```python
from build123d import *

# Parameters (mm, degrees)
SKETCH1_W           = 690.5625
SKETCH1_H           = 320.675
SKETCH1_W_2         = 639.7625
SKETCH1_H_2         = 269.875
SKETCH1_W_3         = 25.4
SKETCH1_W_4         = 79.375
SKETCH1_H_3         = 25.4
BOSS_EXTRUDE1_DEPTH = 617.22
SKETCH2_W           = 566.42
SKETCH2_H           = 269.875
CUT_EXTRUDE1_DEPTH  = 981.137516082
BOSS_EXTRUDE2_DEPTH = 566.42
CUT_EXTRUDE2_REACH  = 741.293
SKETCH6_W           = 566.42
SKETCH6_H           = 79.375
SKETCH7_W           = 127
SKETCH7_H           = 203.2
SKETCH7_W_2         = 261.62
CUT_EXTRUDE3_DEPTH  = 773.950070043
CUT_EXTRUDE4_REACH  = 785.005
SKETCH8_W           = 566.42
SKETCH8_H           = 307.975
CUT_EXTRUDE6_REACH  = 785.005
SKETCH9_W           = 159.433185108
SKETCH9_H           = 305.57390625
SKETCH9_W_2         = 381.586814892
CUT_EXTRUDE8_REACH  = 774.95
SKETCH10_W          = 566.42
SKETCH10_H          = 306.3875
CUT_EXTRUDE10_REACH = 774.95
SKETCH12_W          = 566.42
SKETCH12_H          = 79.375
SKETCH13_W          = 617.22
SKETCH13_H          = 333.375
CUT_EXTRUDE13_DEPTH = 25.4


with BuildPart() as part:
    # Sketch1 → Boss-Extrude1 (new body)
    # profile 1 of 4: a face of its own
    with BuildSketch(Plane(origin=(0, 0, 0), x_dir=(0, 0, -1), z_dir=(1, 0, 0))):
        with Locations((-14.30734375, -160.3375)):
            Rectangle(SKETCH1_W, SKETCH1_H)
        with Locations((-14.30734375, -160.3375)):
            Rectangle(SKETCH1_W_2, SKETCH1_H_2, mode=Mode.SUBTRACT)
    # profile 2 of 4: a face of its own
    with BuildSketch(Plane(origin=(0, 0, 0), x_dir=(0, 0, -1), z_dir=(1, 0, 0))):
        Polygon((-0.81359375, -25.4), (-26.21359375, -25.4), (-26.21359375, -190.5), (-26.21359375, -215.9), (-26.21359375, -295.275), (-0.81359375, -295.275), align=None)
    # profile 3 of 4: a face of its own
    with BuildSketch(Plane(origin=(0, 0, 0), x_dir=(0, 0, -1), z_dir=(1, 0, 0))):
        with Locations((-118.28859375, -160.3375)):
            Rectangle(SKETCH1_W_3, SKETCH1_H_2)
    # profile 4 of 4: a face of its own
    with BuildSketch(Plane(origin=(0, 0, 0), x_dir=(0, 0, -1), z_dir=(1, 0, 0))):
        with Locations((-65.90109375, -203.2)):
            Rectangle(SKETCH1_W_4, SKETCH1_H_3)
    extrude(amount=BOSS_EXTRUDE1_DEPTH)

    # Sketch2 → Cut-Extrude1 (cut, through all)
    with BuildSketch(Plane.XY.offset(359.58859375)):
        with Locations((308.61, -160.3375)):
            Rectangle(SKETCH2_W, SKETCH2_H)
    extrude(amount=-CUT_EXTRUDE1_DEPTH, mode=Mode.SUBTRACT)

    # Sketch4 → Boss-Extrude2 (add)
    with BuildSketch(Plane(origin=(25.4, 0, 0), x_dir=(0, 0, -1), z_dir=(1, 0, 0))):
        Polygon((-26.21359375, -190.5), (-0.81359375, -190.5), (-0.81359375, -215.87774991), (-130.98859375, -215.87774991), (-130.98859375, -190.5), align=None)
    extrude(amount=BOSS_EXTRUDE2_DEPTH)

    # Sketch6 → Cut-Extrude2 (cut, up to next)
    with BuildSketch(Plane(origin=(0, -190.5, 0), x_dir=(1, 0, 0), z_dir=(0, 1, 0)), mode=Mode.PRIVATE) as cut_extrude2_sk1:
        with Locations((308.61, -65.90109375)):
            Rectangle(SKETCH6_W, SKETCH6_H)
    cut_extrude2_tool1 = extrude(cut_extrude2_sk1.sketch, amount=-CUT_EXTRUDE2_REACH, mode=Mode.PRIVATE) & part.part
    add(cut_extrude2_tool1.solids().sort_by_distance((308.61, -190.5, 65.901094))[0], mode=Mode.SUBTRACT)

    # Sketch7 → Cut-Extrude3 (cut, through all)
    with BuildSketch(Plane(origin=(0, -295.275, 0), x_dir=(1, 0, 0), z_dir=(0, 1, 0))):
        with Locations((528.32, -232.58859375)):
            Rectangle(SKETCH7_W, SKETCH7_H)
        with Locations((88.9, -232.58859375)):
            Rectangle(SKETCH7_W, SKETCH7_H)
        with Locations((308.61, -232.58859375)):
            Rectangle(SKETCH7_W_2, SKETCH7_H)
    extrude(amount=-CUT_EXTRUDE3_DEPTH, mode=Mode.SUBTRACT)

    # Sketch8 → Cut-Extrude4 (cut, up to next)
    with BuildSketch(Plane(origin=(0, 0, 0), x_dir=(1, 0, 0), z_dir=(0, 1, 0)), mode=Mode.PRIVATE) as cut_extrude4_sk1:
        with Locations((308.61, -180.20109375)):
            Rectangle(SKETCH8_W, SKETCH8_H)
    cut_extrude4_tool1 = extrude(cut_extrude4_sk1.sketch, amount=-CUT_EXTRUDE4_REACH, mode=Mode.PRIVATE) & part.part
    add(cut_extrude4_tool1.solids().sort_by_distance((308.61, 0, 180.201094))[0], mode=Mode.SUBTRACT)

    # Sketch9 → Cut-Extrude6 (cut, up to next)
    with BuildSketch(Plane(origin=(0, 0, 0), x_dir=(1, 0, 0), z_dir=(0, 1, 0)), mode=Mode.PRIVATE) as cut_extrude6_sk1:
        with Locations((105.116592554, 152.786953125)):
            Rectangle(SKETCH9_W, SKETCH9_H)
    cut_extrude6_tool1 = extrude(cut_extrude6_sk1.sketch, amount=-CUT_EXTRUDE6_REACH, mode=Mode.PRIVATE) & part.part
    # Sketch9 → Cut-Extrude6 (cut, up to next)
    with BuildSketch(Plane(origin=(0, 0, 0), x_dir=(1, 0, 0), z_dir=(0, 1, 0)), mode=Mode.PRIVATE) as cut_extrude6_sk2:
        with Locations((401.026592554, 152.786953125)):
            Rectangle(SKETCH9_W_2, SKETCH9_H)
    cut_extrude6_tool2 = extrude(cut_extrude6_sk2.sketch, amount=-CUT_EXTRUDE6_REACH, mode=Mode.PRIVATE) & part.part
    add(cut_extrude6_tool1.solids().sort_by_distance((105.116593, 0, -152.786953))[0], mode=Mode.SUBTRACT)
    add(cut_extrude6_tool2.solids().sort_by_distance((401.026593, 0, -152.786953))[0], mode=Mode.SUBTRACT)

    # Sketch10 → Cut-Extrude8 (cut, up to next)
    with BuildSketch(Plane(origin=(0, -295.275, 0), x_dir=(1, 0, 0), z_dir=(0, 1, 0)), mode=Mode.PRIVATE) as cut_extrude8_sk1:
        with Locations((308.61, 152.38015625)):
            Rectangle(SKETCH10_W, SKETCH10_H)
    cut_extrude8_tool1 = extrude(cut_extrude8_sk1.sketch, amount=-CUT_EXTRUDE8_REACH, mode=Mode.PRIVATE) & part.part
    add(cut_extrude8_tool1.solids().sort_by_distance((308.61, -295.275, -152.380156))[0], mode=Mode.SUBTRACT)

    # Sketch12 → Cut-Extrude10 (cut, up to next)
    with BuildSketch(Plane(origin=(0, -295.275, 0), x_dir=(1, 0, 0), z_dir=(0, 1, 0)), mode=Mode.PRIVATE) as cut_extrude10_sk1:
        with Locations((308.61, -65.90109375)):
            Rectangle(SKETCH12_W, SKETCH12_H)
    cut_extrude10_tool1 = extrude(cut_extrude10_sk1.sketch, amount=-CUT_EXTRUDE10_REACH, mode=Mode.PRIVATE) & part.part
    add(cut_extrude10_tool1.solids().sort_by_distance((308.61, -295.275, 65.901094))[0], mode=Mode.SUBTRACT)

    # Sketch13 → Cut-Extrude13 (cut)
    with BuildSketch(Plane(origin=(0, 0, 0), x_dir=(1, 0, 0), z_dir=(0, 1, 0))):
        with Locations((308.61, -192.90109375)):
            Rectangle(SKETCH13_W, SKETCH13_H)
    extrude(amount=-CUT_EXTRUDE13_DEPTH, mode=Mode.SUBTRACT)


solid = part.part
```
Check sheet for the modelled part. Datum: model origin and axes. Units: mm. A direction names the side the tool comes from. Coordinates: 2 decimals unless noted, no trailing zeros. Loops run counter-clockwise (first coordinate to the right, second up) from the corner with the lowest first, then second, coordinate; pieces in that order, holes last.
1) Sectioned sample at A-A (z = -153). Record the boundary of the cut face in (x, y) (3 decimals).
2) Access from +Z, -Z, +X, -X, +Y, -Y to the whole of each face (thin tool, end or side, straight path). Record for faces 1 (the face through (184.833, -13, -151)), 2 (the face through (591.82, -207, 67)), 3 (the face through (604, -295.275, 66)).
3) Sectioned sample at B-B (y = -155). Count the separate pieces of the cut face and the enclosed holes in it, and give its area (3 significant figures).
4) Gauge pin test, flat end, axial feed: pin 1 (12.5 mm diameter, centred on x = 16.5, z = 74.5, fed in from +Y). Record the tip position at first contact, or that the pin passes through.
5) Release check for a two-part mould opening along Z. For faces 4 (the face through (591.82, -308, 234)), 5 (the face through (604, -162, -305.574)), 6 (the face through (13, -25.4, 118)) record: released by +Z, released by -Z, zero draft, split by the parting line, or undercut.
6) Sectioned sample at C-C (z = 95.5). Record the boundary of the cut face in (x, y) (3 decimals).
7) Material ranges on probe 1 along Z at (x, y) = (360, -299); probe 2 along Z at (x, y) = (29.5, -197.5); probe 3 along Y at (x, z) = (438, 22) (3 decimals), recorded low to high.
Check sheet entries:
1. outline: (0, -320.675) - (25.4, -320.675) - (25.4, -295.275) - (0, -295.275) - close; (0, -25.4) - (25.4, -25.4) - (25.4, 0) - (0, 0) - close; (184.833, -25.4) - (210.233, -25.4) - (210.233, 0) - (184.833, 0) - close; (591.82, -320.675) - (617.22, -320.675) - (617.22, -295.275) - (591.82, -295.275) - close; (591.82, -25.4) - (617.22, -25.4) - (617.22, 0) - (591.82, 0) - close
2. face 1: +Y, -Y
2. face 2: none
2. face 3: +X, -X
3. separate pieces: 8
3. enclosed holes: 0
3. area: 5,160 mm2
4. pin 1: stops at y = -190.5
5. face 4: undercut
5. face 5: undercut
5. face 6: zero draft
6. outline: (0, -320.675) - (25.4, -320.675) - (25.4, -295.275) - (0, -295.275) - close; (0, -215.9) - (25.4, -215.9) - (25.4, -190.5) - (0, -190.5) - close; (591.82, -320.675) - (617.22, -320.675) - (617.22, -295.275) - (591.82, -295.275) - close; (591.82, -215.9) - (617.22, -215.9) - (617.22, -190.5) - (591.82, -190.5) - close
7. probe 1: z = -330.97 to -305.57, 0.81 to 26.21, 105.59 to 130.99, 334.19 to 359.59
7. probe 2: z = 0.81 to 26.21, 105.59 to 130.99
7. probe 3: y = -320.675 to -295.275, -215.878 to -190.5, -25.4 to 0
